For this review, take the finished solid that the model builds, in its own axes (mm). A direction names the side the tool comes from. Give positions to 0.01 mm unless a question says otherwise; leave off trailing zeros. Order: outer loops, then holes, each group sorted by start corner. A loop starts at its lowest first (then second) coordinate and runs counter-clockwise, first axis right, second up. Notation, with made-up numbers: (-36, 6.25) - (-1, 6.25) arc R22 cw to (-1, 17.25) - close; hole circle Ø2 at (9.25, -30.5). An arc over 180 degrees is marked (long way). One line per item, written item: value.
```python
from build123d import *

# Parameters (mm, degrees)
SKETCH_W        = 54.3
SKETCH_H        = 38
PAD_DEPTH       = 2
SKETCH001_W     = 54.3
SKETCH001_H     = 2
PAD001_DEPTH    = 22
SKETCH002_R     = 2.45
PAD002_DEPTH    = 5
SKETCH003_W     = 40
SKETCH003_H     = 22
PAD003_DEPTH    = 2
SKETCH004_W     = 40
SKETCH004_H     = 22
PAD004_DEPTH    = 2
SKETCH005_W     = 6.85
SKETCH005_H     = 15
PAD005_DEPTH    = 8
SKETCH006_R     = 1.4
POCKET_DEPTH    = 15
FILLET_R        = 3
FILLET001_R     = 2
SKETCH007_W     = 6.85
SKETCH007_H     = 25.8
PAD006_DEPTH    = 20
SKETCH008_R     = 1.4
POCKET001_DEPTH = 15
PAD007_DEPTH    = 2
SKETCH010_R     = 1.4
PAD008_DEPTH    = 2
SKETCH011_R     = 1.4
PAD009_DEPTH    = 2
FILLET002_R     = 1
FILLET003_R     = 1
FILLET004_R     = 1
FILLET005_R     = 1
FILLET006_R     = 1


with BuildPart() as part:
    # Sketch → Pad (new body)
    with BuildSketch(Plane.XY):
        with Locations((27.15, 21)):
            Rectangle(SKETCH_W, SKETCH_H)
    extrude(amount=PAD_DEPTH)

    # Sketch001 → Pad001 (join)
    with BuildSketch(Plane.XY):
        with Locations((27.15, 1)):
            Rectangle(SKETCH001_W, SKETCH001_H)
    extrude(amount=PAD001_DEPTH)

    # Sketch002 → Pad002 (join)
    with BuildSketch(Plane.XZ):
        with Locations((37.25, 12)):
            Circle(SKETCH002_R)
    extrude(amount=PAD002_DEPTH)

    # Sketch003 (on Face2 of Pad002) → Pad003 (join)
    with BuildSketch(Plane(origin=(0, 0, 0), x_dir=(0, -1, 0), z_dir=(-1, 0, 0))):
        with Locations((-20, 11)):
            Rectangle(SKETCH003_W, SKETCH003_H)
    extrude(amount=PAD003_DEPTH)

    # Sketch004 (on Face3 of Pad003) → Pad004 (join)
    with BuildSketch(Plane.YZ.offset(54.3)):
        with Locations((20, 11)):
            Rectangle(SKETCH004_W, SKETCH004_H)
    extrude(amount=PAD004_DEPTH)

    # Sketch005 (on Face5 of Pad004) → Pad005 (join)
    with BuildSketch(Plane.XY.offset(2)):
        with Locations((50.875, 20.3)):
            Rectangle(SKETCH005_W, SKETCH005_H)
    extrude(amount=PAD005_DEPTH)

    # Sketch006 (on Face15 of Pad005) → Pocket (cut)
    with BuildSketch(Plane(origin=(0, 27.8, 0), x_dir=(-1, 0, 0), z_dir=(0, 1, 0))):
        with Locations((-51.3, 7)):
            Circle(SKETCH006_R)
    extrude(amount=-POCKET_DEPTH, mode=Mode.SUBTRACT)

    # Fillet
    fillet_edges = [part.edges().sort_by_distance(p)[0] for p in [
        (47.45, 20.3, 10),
    ]]
    fillet(fillet_edges, radius=FILLET_R)

    # Fillet001
    fillet001_edges = [part.edges().sort_by_distance(p)[0] for p in [
        (52.375, 12.8, 10),
    ]]
    fillet(fillet001_edges, radius=FILLET001_R)

    # Sketch007 (on Face5 of Fillet001) → Pad006 (join)
    with BuildSketch(Plane.XY.offset(2)):
        with Locations((3.425, 14.9)):
            Rectangle(SKETCH007_W, SKETCH007_H)
    extrude(amount=PAD006_DEPTH)

    # Sketch008 (on Face14 of Pad006) → Pocket001 (cut)
    with BuildSketch(Plane(origin=(0, 27.8, 0), x_dir=(-1, 0, 0), z_dir=(0, 1, 0))):
        with Locations((-3, 7)):
            Circle(SKETCH008_R)
        with Locations((-3, 17)):
            Circle(SKETCH008_R)
    extrude(amount=-POCKET001_DEPTH, mode=Mode.SUBTRACT)

    # Sketch009 (on Face21 of Pocket001) → Pad007 (join)
    with BuildSketch(Plane.XY.offset(22)):
        Polygon((54.3, 2), (54.3, 40), (56.3, 40), (56.3, 0), (-2, 0), (-2, 40), (6.85, 40), (6.85, 2), align=None)
    extrude(amount=PAD007_DEPTH)

    # Sketch010 (on Face22 of Pad007) → Pad008 (join)
    with BuildSketch(Plane.YZ.offset(6.85)):
        with BuildLine():
            Line((2, 24), (38, 24))
            Line((38, 29), (38, 24))
            ThreePointArc((38, 29), (37.326745, 31.511013), (35.487593, 33.348396))
            Line((35.487593, 33.348396), (9.497223, 48.331729))
            ThreePointArc((9.497223, 48.331729), (4.498612, 48.329325), (2, 44))
            Line((2, 44), (2, 24))
        make_face()
        with Locations((7, 44)):
            Circle(SKETCH010_R, mode=Mode.SUBTRACT)
        with Locations((32.980762, 29)):
            Circle(SKETCH010_R, mode=Mode.SUBTRACT)
    extrude(amount=-PAD008_DEPTH)

    # Sketch011 (on Face20 of Pad008) → Pad009 (join)
    with BuildSketch(Plane(origin=(54.3, 0, 0), x_dir=(0, -1, 0), z_dir=(-1, 0, 0))):
        with BuildLine():
            Line((-38, 24), (-38, 29))
            ThreePointArc((-35.487593, 33.348396), (-37.326745, 31.511013), (-38, 29))
            Line((-35.487593, 33.348396), (-9.497223, 48.331729))
            ThreePointArc((-2, 44), (-4.498612, 48.329325), (-9.497223, 48.331729))
            Line((-2, 44), (-2, 24))
            Line((-2, 24), (-38, 24))
        make_face()
        with Locations((-7, 44)):
            Circle(SKETCH011_R, mode=Mode.SUBTRACT)
        with Locations((-32.980762, 29)):
            Circle(SKETCH011_R, mode=Mode.SUBTRACT)
    extrude(amount=-PAD009_DEPTH)

    # Fillet002
    fillet002_edges = [part.edges().sort_by_distance(p)[0] for p in [
        (-2, 20, 0),
    ]]
    fillet(fillet002_edges, radius=FILLET002_R)

    # Fillet003
    fillet003_edges = [part.edges().sort_by_distance(p)[0] for p in [
        (27.15, 0, 0),
    ]]
    fillet(fillet003_edges, radius=FILLET003_R)

    # Fillet004
    fillet004_edges = [part.edges().sort_by_distance(p)[0] for p in [
        (27.15, 40, 0),
    ]]
    fillet(fillet004_edges, radius=FILLET004_R)

    # Fillet005
    fillet005_edges = [part.edges().sort_by_distance(p)[0] for p in [
        (56.3, 20, 0),
    ]]
    fillet(fillet005_edges, radius=FILLET005_R)

    # Fillet006
    fillet006_edges = [part.edges().sort_by_distance(p)[0] for p in [
        (27.15, 0, 24),
    ]]
    fillet(fillet006_edges, radius=FILLET006_R)


solid = part.part
```
(1) Take a section at D-D (y = 23). Write out the cut boundary in (x, z), then the cut area to 3 significant figures.
Answers below:
outline: (-2, 1) arc R1 ccw to (-1, 0) - (55.3, 0) arc R1 ccw to (56.3, 1) - (56.3, 40.55) - (54.3, 40.55) - (54.3, 10) - (50.45, 10) arc R3 ccw to (47.45, 7) - (47.45, 2) - (6.85, 2) - (6.85, 40.55) - (4.85, 40.55) - (4.85, 24) - (-1, 24) arc R1 ccw to (-2, 23) - close; hole circle Ø2.8 at (3, 7); hole circle Ø2.8 at (3, 17); hole circle Ø2.8 at (51.3, 7)
area: 455 mm^2
(2) Take a section at B-B (y = 7.5). Write out the cut boundary in (x, z), then the cut area to 3 significant figures.
Answers below:
outline: (-2, 1) arc R1 ccw to (-1, 0) - (55.3, 0) arc R1 ccw to (56.3, 1) - (56.3, 42.69) - (54.3, 42.69) - (54.3, 2) - (6.85, 2) - (6.85, 42.69) - (4.85, 42.69) - (4.85, 24) - (-1, 24) arc R1 ccw to (-2, 23) - close; (4.85, 45.31) - (6.85, 45.31) - (6.85, 48.97) - (4.85, 48.97) - close; (54.3, 45.31) - (56.3, 45.31) - (56.3, 48.97) - (54.3, 48.97) - close
area: 444 mm^2
(3) Machinability: for faces 5 (the face through (3, 27.8, 12)), 6 (the face through (48.02, 13.4, 4.54)), 7 (the face through (48.35, 21.39, 9.14)), which of the approach directions +Z, -Z, +X, -X, +Y, -Y give a long, thin tool a straight path to every point of the face, cutting with its end or side? Answer none if there is none.
Answers below:
face 5: +Y
face 6: +Z
face 7: +Z, +Y
(4) Wall thickness on line 1 (Z direction, x = 3, y = 23.5); line 2 (Z direction, x = 5.85, y = 7); line 3 (X direction, y = 18, z = 38): over which ranges is each line inside the solid? List them lowest first. Write a range as from..to.
Answers below:
line 1: z = 0..5.6, 8.4..15.6, 18.4..24
line 2: z = 0..42.6, 45.4..49
line 3: x = 4.85..6.85, 54.3..56.3
(5) Take a section at C-C (x = 19). Write out the cut boundary in (y, z).
Answers below:
outline: (0, 1) arc R1 ccw to (1, 0) - (39, 0) arc R1 ccw to (40, 1) - (40, 2) - (2, 2) - (2, 24) - (1, 24) arc R1 ccw to (0, 23) - close
(6) For P1, Ø19, axis at x = 35.5, y = 18, coming from the +Z side; P2, Ø1.4, axis at x = 3, z = 7.5, coming from the +Y side; P3, Ø3.5, axis at x = 51.3, z = 7, coming from the -Y side, all flat-tipped, find the tip position at first contact; note any pin that passes through.
Answers below:
P1: stops at z = 2
P2: stops at y = 12.8
P3: stops at y = 0
(7) Take a section at A-A (z = 12). Write out the cut boundary in (x, y), then the cut area to 3 significant figures.
Answers below:
outline: (-2, 1) arc R1 ccw to (-1, 0) - (34.8, 0) - (34.8, -5) - (39.7, -5) - (39.7, 0) - (55.3, 0) arc R1 ccw to (56.3, 1) - (56.3, 39) arc R1 ccw to (55.3, 40) - (54.3, 40) - (54.3, 2) - (6.85, 2) - (6.85, 27.8) - (0, 27.8) - (0, 40) - (-1, 40) arc R1 ccw to (-2, 39) - close
area: 469 mm^2
(8) Draft analysis for pull direction Z (two halves, no side actions). For faces 1 (the face through (56.3, 20, 20)), 2 (the face through (5.86, 32.8, 30.39)), 3 (the face through (39.587, -2.465, 12.736)), 4 (the face through (55.29, 37.31, 31.54)), state which applies: pulls with the +Z half, pulls with the -Z half, needs draft (parallel to the pull), parting line crosses it, or undercut.
Answers below:
face 1: needs draft
face 2: undercut
face 3: parting line crosses it
face 4: pulls with the +Z half
